Model file for the job. Use its own axes, mm. A direction names the side the tool comes from. Round coordinates to 2 decimals unless told otherwise and drop trailing zeros. Order: outer loops, then holes, each group sorted by start corner. A loop starts at its lowest first (then second) coordinate and runs counter-clockwise, first axis right, second up. Notation, with made-up numbers: (65, -4.75) - (76, -4.75) arc R14 ccw to (76, 13.25) - close; hole circle Ø10 at (0.5, 55). An arc over 180 degrees is marked (long way). Write item = value, one per line.
Autodesk Inventor part; units mm, degrees
ref_plane "YZ Plane" through (0, 0, 0) normal (1, 0, 0) x (0, 1, 0)
ref_plane "XZ Plane" through (0, 0, 0) normal (0, 1, 0) x (-1, 0, 0)
ref_plane "XY Plane" through (0, 0, 0) normal (0, 0, 1) x (1, 0, 0)
sketch "Sketch1" plane through (0, 0, 0) normal (0, 0, 1) x (1, 0, 0)
  line L0 (0, 0) -> (40, 0)
  line L1 (40, 0) -> (40, 30)
  line L2 (0, 0) -> (-40, 0)
  line L3 (-40, 0) -> (-40, 30)
  arc A0 (-22.225, 60) -> (-40, 30) centre (-10.109, 32.5554) ccw
  arc A1 (40, 30) -> (20, 60) centre (10.0481, 31.6988) ccw
  line L4 (-22.225, 60) -> (-18.1866, 55.5625)
  line L5 (20, 60) -> (15.875, 55.5625)
  line L6 (-18.1866, 55.5625) -> (15.875, 55.5625)
  circle A2 centre (0, 0) radius 11.25
  point P0 (0, 20)
  point P1 (-11.25, 0)
  point P2 (11.25, 0)
  dimension "d0" = 40
  dimension "d1" = 30
  dimension "d2" = 40
  dimension "d3" = 30
  dimension "d4" = 30
  dimension "d5" = 60
  dimension "d7" = 6
  dimension "d9" = 20
  dimension "d10" = 22.5
extrude "Extrusion1" add sketch "Sketch1" along normal blind 228.6 contours A2 L2 L3 A0 L4 L6 L5 A1 L1 L0
properties part number "arm rest final 1"
1) Wall check: line 1 along X through (y, z) = (24, 123); line 2 along Y through (x, z) = (-15, 41.5); line 3 along X through (y, z) = (3.5, 93). Give the ranges that are in metal, low to high.
Conclusion:
line_1 = -40 to 40
line_2 = 0 to 55.56
line_3 = -40 to -10.69, 10.69 to 40
2) Cut at B-B (x = 13.5). Write the cut outline in (y, z), and give its area (3 significant figures).
Conclusion:
outline = (0, 0) - (55.56, 0) - (55.56, 228.6) - (0, 228.6) - close
area = 12,700 mm^2
3) Cut at C-C (y = 42). Write the cut outline in (x, z).
Conclusion:
outline = (-38.58, 0) - (38.22, 0) - (38.22, 228.6) - (-38.58, 228.6) - close
4) Flat gauge pins, fed straight in: pin 1 Ø6 at (x, z) = (-12.5, 196) entering from +Y; pin 2 Ø15 at (y, z) = (20, 65.5) entering from -X; pin 3 Ø1 at (y, z) = (22, 124) entering from +X. Where does each tip first touch, or does it go through?
Conclusion:
pin_1 = 55.56
pin_2 = -40
pin_3 = 40
5) Mould opens along X. For faces 1 (the face through (-1, 55.562, 113)), 2 (the face through (-25, 0, 113)), 3 (the face through (40, 15, 113)), 4 (the face through (-40, 15, 113)) say: +X half, -X half, draft (parallel to the pull), parting line (faces both ways), or undercut.
Conclusion:
face_1 = undercut
face_2 = draft
face_3 = +X half
face_4 = -X half
6) 3-axis set-ups, long thin cutter, end or side, ignore diameter. For faces 5 (the face through (-0.247, 11.247, 112.7)), 6 (the face through (-20.23, 57.81, 112.7)): which of +Z, -Z, +X, -X, +Y, -Y reach the whole face in a straight line?
Conclusion:
face_5 = +Z, -Z, -Y
face_6 = +Z, -Z, +Y
